```python
from build123d import *

# Parameters (mm, degrees)
F1_DEPTH = 4


with BuildPart() as f1:
    # F0 (on Top) → F1 (new body)
    with BuildSketch(Plane.XY):
        with BuildLine():
            ThreePointArc((4.898979, -1), (4.974681, -0.502545), (5, 0))
            ThreePointArc((5, 0), (4.974681, 0.502545), (4.898979, 1))
            ThreePointArc((4.898979, 1), (4.829629, 1.294095), (4.742641, 1.583464))
            ThreePointArc((4.742641, 1.583464), (4.330127, 2.5), (3.742641, 3.315515))
            ThreePointArc((3.742641, 3.315515), (3.535534, 3.535534), (3.315515, 3.742641))
            ThreePointArc((3.315515, 3.742641), (2.5, 4.330127), (1.583464, 4.742641))
            ThreePointArc((1.583464, 4.742641), (1.294095, 4.829629), (1, 4.898979))
            Line((1, 4.898979), (-1, 4.898979))
            ThreePointArc((-1, 4.898979), (-1.294095, 4.829629), (-1.583464, 4.742641))
            ThreePointArc((-1.583464, 4.742641), (-2.5, 4.330127), (-3.315515, 3.742641))
            ThreePointArc((-3.315515, 3.742641), (-3.535534, 3.535534), (-3.742641, 3.315515))
            ThreePointArc((-3.742641, 3.315515), (-4.330127, 2.5), (-4.742641, 1.583464))
            ThreePointArc((-4.742641, 1.583464), (-4.829629, 1.294095), (-4.898979, 1))
            ThreePointArc((-4.898979, 1), (-5, 0), (-4.898979, -1))
            ThreePointArc((-4.898979, -1), (-4.829629, -1.294095), (-4.742641, -1.583464))
            ThreePointArc((-4.742641, -1.583464), (-4.330127, -2.5), (-3.742641, -3.315515))
            ThreePointArc((-3.742641, -3.315515), (-3.535534, -3.535534), (-3.315515, -3.742641))
            ThreePointArc((-3.315515, -3.742641), (-2.5, -4.330127), (-1.583464, -4.742641))
            ThreePointArc((-1.583464, -4.742641), (-1.294095, -4.829629), (-1, -4.898979))
            ThreePointArc((-1, -4.898979), (0, -5), (1, -4.898979))
            ThreePointArc((1, -4.898979), (1.294095, -4.829629), (1.583464, -4.742641))
            ThreePointArc((1.583464, -4.742641), (2.5, -4.330127), (3.315515, -3.742641))
            ThreePointArc((3.315515, -3.742641), (3.535534, -3.535534), (3.742641, -3.315515))
            ThreePointArc((3.742641, -3.315515), (4.330127, -2.5), (4.742641, -1.583464))
            ThreePointArc((4.742641, -1.583464), (4.829629, -1.294095), (4.898979, -1))
        make_face()
        with BuildLine():
            Line((-1, 4.898979), (1, 4.898979))
            ThreePointArc((1, 4.898979), (0, 5), (-1, 4.898979))
        make_face()
        with BuildLine():
            ThreePointArc((-3.315515, 3.742641), (-2.5, 4.330127), (-1.583464, 4.742641))
            Line((-1.583464, 4.742641), (-2.94949, 5.108666))
            Line((-2.94949, 5.108666), (-3.315515, 3.742641))
        make_face()
        with BuildLine():
            ThreePointArc((-1, 4.898979), (0, 5), (1, 4.898979))
            Line((1, 4.898979), (0, 5.898979))
            Line((0, 5.898979), (-1, 4.898979))
        make_face()
        with BuildLine():
            ThreePointArc((1.583464, 4.742641), (2.5, 4.330127), (3.315515, 3.742641))
            Line((3.315515, 3.742641), (2.94949, 5.108666))
            Line((2.94949, 5.108666), (1.583464, 4.742641))
        make_face()
        with BuildLine():
            ThreePointArc((3.742641, 3.315515), (4.330127, 2.5), (4.742641, 1.583464))
            Line((4.742641, 1.583464), (5.108666, 2.94949))
            Line((5.108666, 2.94949), (3.742641, 3.315515))
        make_face()
        with BuildLine():
            ThreePointArc((4.898979, 1), (4.974681, 0.502545), (5, 0))
            ThreePointArc((5, 0), (4.974681, -0.502545), (4.898979, -1))
            Line((4.898979, -1), (5.898979, 0))
            Line((5.898979, 0), (4.898979, 1))
        make_face()
        with BuildLine():
            Line((5.108666, -2.94949), (4.742641, -1.583464))
            ThreePointArc((4.742641, -1.583464), (4.330127, -2.5), (3.742641, -3.315515))
            Line((3.742641, -3.315515), (5.108666, -2.94949))
        make_face()
        with BuildLine():
            Line((2.94949, -5.108666), (3.315515, -3.742641))
            ThreePointArc((3.315515, -3.742641), (2.5, -4.330127), (1.583464, -4.742641))
            Line((1.583464, -4.742641), (2.94949, -5.108666))
        make_face()
        with BuildLine():
            Line((0, -5.898979), (1, -4.898979))
            ThreePointArc((1, -4.898979), (0, -5), (-1, -4.898979))
            Line((-1, -4.898979), (0, -5.898979))
        make_face()
        with BuildLine():
            Line((-2.94949, -5.108666), (-1.583464, -4.742641))
            ThreePointArc((-1.583464, -4.742641), (-2.5, -4.330127), (-3.315515, -3.742641))
            Line((-3.315515, -3.742641), (-2.94949, -5.108666))
        make_face()
        with BuildLine():
            Line((-5.108666, -2.94949), (-3.742641, -3.315515))
            ThreePointArc((-3.742641, -3.315515), (-4.330127, -2.5), (-4.742641, -1.583464))
            Line((-4.742641, -1.583464), (-5.108666, -2.94949))
        make_face()
        with BuildLine():
            ThreePointArc((-4.898979, -1), (-5, 0), (-4.898979, 1))
            Line((-4.898979, 1), (-5.898979, 0))
            Line((-5.898979, 0), (-4.898979, -1))
        make_face()
        with BuildLine():
            ThreePointArc((-4.742641, 1.583464), (-4.330127, 2.5), (-3.742641, 3.315515))
            Line((-3.742641, 3.315515), (-5.108666, 2.94949))
            Line((-5.108666, 2.94949), (-4.742641, 1.583464))
        make_face()
    extrude(amount=F1_DEPTH)


solid = f1.part
```
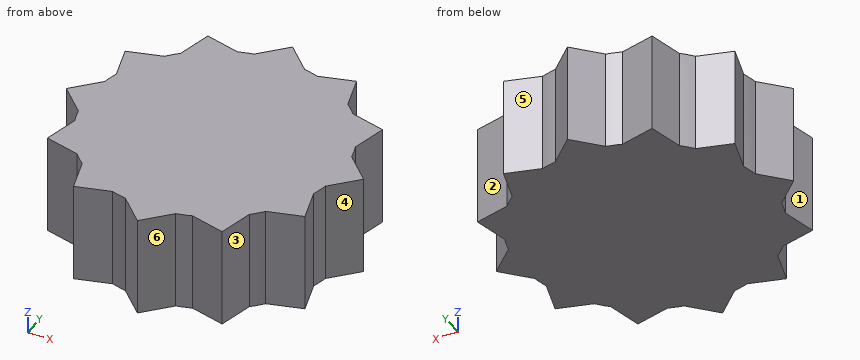
Could you check a few things on this model? Use its own coordinates, in mm. Face numbers are marked on the shaded views. A direction names the side the tool comes from. Round coordinates to 2 decimals unless told otherwise and drop trailing zeros. Loops run counter-clockwise (first coordinate to the right, second up) from the corner with the lowest first, then second, coordinate; pieces in that order, holes last. Notation, with made-up numbers: (87.5, 24) - (128.5, 24) arc R25 ccw to (128.5, 45) - close; hole circle Ø9 at (84, 65). An arc over 180 degrees is marked (long way). Use CSV: the item, a comma, the result in double quotes.
Item 1: If we section it at A-A on y = 4: List the corners of the cut face in (x, z) for me.
Here are the results:
outline,"(-3.25, 0) - (3.25, 0) - (3.25, 4) - (-3.25, 4) - close"
Item 2: If we mould it in two halves opening along Y, with no side actions, what happens to the marked faces 1, 2 and 3? For each: pulls with the +Y half, pulls with the -Y half, needs draft (parallel to the pull), parting line crosses it, or undercut.
Here are the results:
face 1,"undercut"
face 2,"pulls with the +Y half"
face 3,"pulls with the -Y half"
Item 3: For the marked faces 4, 5 and 6, which set-ups out of +Z, -Z, +X, -X, +Y, -Y let a thin tool reach every point of the face, with its end or its side?
Here are the results:
face 4,"+Z, -Z, +X"
face 5,"+Z, -Z, +Y"
face 6,"+Z, -Z, -Y"
Item 4: I need wall thicknesses on L1, parallel to X at y = -2.75, z = 1.1; L2, parallel to X at y = 4, z = 3.35; L3, parallel to Y at x = 4.5, z = 1.8. Which ranges of each line are inside material? Lowest first, please. Write a range as [from, to].
Here are the results:
L1,"x = [-5.06, 5.06]"
L2,"x = [-3.25, 3.25]"
L3,"y = [-3.11, 3.11]"
Item 5: If we section it at B-B on x = -0.25: List the corners of the cut face in (y, z) for me.
Here are the results:
outline,"(-5.65, 0) - (5.65, 0) - (5.65, 4) - (-5.65, 4) - close"
